Can you work these out from the model? Positions are in its coordinate system, mm. A direction names the side the tool comes from. Give positions to 0.01 mm unless a question says otherwise; leave off trailing zeros. Write each loop counter-clockwise with the first axis right and the second up, starting at its lowest first coordinate (ties: lowest second). Pieces come first, ordered by that corner, then holes.
```python
from build123d import *

# Parameters (mm, degrees)
F0_R     = 2.5
F1_DEPTH = 12.7
F0_R_2   = 4
F2_DEPTH = 8.2
F0_R_3   = 5
F3_DEPTH = 2
F5_D     = 2
F5_DEPTH = 3
F5_TIP   = 0.600860619


with BuildPart() as f1:
    # F0 (on Top) → F1 (new body)
    with BuildSketch(Plane.XY):
        Circle(F0_R)
    extrude(amount=F1_DEPTH)

    # F0 (on Top) → F2 (join)
    with BuildSketch(Plane.XY):
        Circle(F0_R_2)
        Circle(F0_R, mode=Mode.SUBTRACT)
    extrude(amount=F2_DEPTH)

    # F0 (on Top) → F3 (join)
    with BuildSketch(Plane.XY):
        Circle(F0_R_3)
        Circle(F0_R_2, mode=Mode.SUBTRACT)
    extrude(amount=F3_DEPTH)

    # F5
    with Locations(Plane.XY.offset(12.7)):
        with Locations((0, 0)):
            Hole(F5_D / 2, depth=F5_DEPTH)
            with Locations((0, 0, -(F5_DEPTH + F5_TIP / 2))):  # 118° drill point
                Cone(0, F5_D / 2, F5_TIP, mode=Mode.SUBTRACT)


solid = f1.part
```
1) Please list where these lines run through material, in increasing order: L1, parallel to Y at x = 0, z = 10.95; L2, parallel to Z at x = 3.75, y = -0.5; L3, parallel to Z at x = 0.5, y = -4.25.
Values follow:
L1: y = -2.5 to -1, 1 to 2.5
L2: z = 0 to 8.2
L3: z = 0 to 2
2) Suppose I cut it at C-C on x = -1.25. Write out the boundary of the cut face in (y, z), plus the area to 3 significant figures.
Values follow:
outline: (-4.84, 0) - (4.84, 0) - (4.84, 2) - (3.8, 2) - (3.8, 8.2) - (2.17, 8.2) - (2.17, 12.7) - (-2.17, 12.7) - (-2.17, 8.2) - (-3.8, 8.2) - (-3.8, 2) - (-4.84, 2) - close
area: 86.0 mm2
3) For faces 1 (the face through (1, -1, 12.7)), 2 (the face through (0, -1, 11)), which set-ups out of +Z, -Z, +X, -X, +Y, -Y let a thin tool reach every point of the face, with its end or its side?
Values follow:
face 1: +Z, +X, -X, +Y, -Y
face 2: +Z
4) For pin 1 Ø3 at (x, z) = (-2.5, 5) entering from +Y; pin 2 Ø3 at (y, z) = (-2, 5) entering from +X; pin 3 Ø3 at (y, z) = (-3.5, 7) entering from +X, each with a flat end and sliding along its axis, tell me the tip position at first contact or that it passes through.
Values follow:
pin 1: stops at y = 3.87
pin 2: stops at x = 3.97
pin 3: stops at x = 3.46
5) If we mould it in two halves opening along Y, with no side actions, what happens to faces 3 (the face through (0, 0, 0)), 4 (the face through (-0.867, -3.905, 5.057)), 5 (the face through (-0.038, -0.17, 9.203))? For each: +Y half, -Y half, draft (parallel to the pull), parting line (faces both ways), or undercut.
Values follow:
face 3: draft
face 4: parting line
face 5: undercut
6) Suppose I cut it at A-A on y = 3.75. Write out the boundary of the cut face in (x, z), plus the area to 3 significant figures.
Values follow:
outline: (-3.31, 0) - (3.31, 0) - (3.31, 2) - (1.39, 2) - (1.39, 8.2) - (-1.39, 8.2) - (-1.39, 2) - (-3.31, 2) - close
area: 30.5 mm2
7) Suppose I cut it at B-B on z = 5.75. Write out the boundary of the cut face in (x, y), plus the area to 3 significant figures.
Values follow:
outline: circle Ø8 at (0, 0)
area: 50.3 mm2
8) Suppose I cut it at D-D on y = -2. Write out the boundary of the cut face in (x, z).
Values follow:
outline: (-4.58, 0) - (4.58, 0) - (4.58, 2) - (3.46, 2) - (3.46, 8.2) - (1.5, 8.2) - (1.5, 12.7) - (-1.5, 12.7) - (-1.5, 8.2) - (-3.46, 8.2) - (-3.46, 2) - (-4.58, 2) - close
